```python
from build123d import *

# Parameters (mm, degrees)
F0_W     = 412.75
F0_H     = 295.275
F1_DEPTH = 25.4
F2_W     = 19.05
F2_H     = 387.35
F3_DEPTH = 25.4


with BuildPart() as f1:
    # F0 (on Top) → F1 (new body)
    with BuildSketch(Plane.XY):
        Polygon((279.4, -203.2), (279.4, 203.2), (-279.4, 203.2), (-330.2, 203.2), (-330.2, -203.2), (-279.4, -203.2), align=None)
        Rectangle(F0_W, F0_H, mode=Mode.SUBTRACT)
    extrude(amount=F1_DEPTH)

    # F2 (on face) → F3 (join)
    with BuildSketch(Plane(origin=(0, 0, 0), x_dir=(1, 0, 0), z_dir=(0, 0, -1))):
        Polygon((279.4, 203.2), (-330.2, 203.2), (-330.2, 184.15), (-311.15, 184.15), (260.35, 184.15), (279.4, 184.15), align=None)
        with Locations((269.875, -9.525)):
            Rectangle(F2_W, F2_H)
        with Locations((-320.675, -9.525)):
            Rectangle(F2_W, F2_H)
    extrude(amount=F3_DEPTH)


solid = f1.part
```
CAD build for the part. Positions are in the model's coordinates, mm. A direction names the side the tool comes from. Round coordinates to 2 decimals unless told otherwise and drop trailing zeros. Write each loop counter-clockwise with the first axis right and the second up, starting at its lowest first coordinate (ties: lowest second). Pieces come first, ordered by that corner, then holes.
Item 1: Band-saw the part on A-A on y = 0.5. Write the cut outline in (x, z) (3 decimals).
Filled in:
outline: (-330.2, -25.4) - (-311.15, -25.4) - (-311.15, 0) - (-206.375, 0) - (-206.375, 25.4) - (-330.2, 25.4) - close; (206.375, 0) - (260.35, 0) - (260.35, -25.4) - (279.4, -25.4) - (279.4, 25.4) - (206.375, 25.4) - close
Item 2: Band-saw the part on B-B on x = 80.5. Write the cut outline in (y, z).
Filled in:
outline: (-203.2, -25.4) - (-184.15, -25.4) - (-184.15, 0) - (-147.64, 0) - (-147.64, 25.4) - (-203.2, 25.4) - close; (147.64, 0) - (203.2, 0) - (203.2, 25.4) - (147.64, 25.4) - close
Item 3: Drill centre lines: L1, parallel to X at y = 132, z = -14.5; L2, parallel to X at y = 80.5, z = 19 (3 decimals); L3, parallel to Y at x = 199, z = 3.5. Where is each one in solid material? Low to high.
Filled in:
L1: x = -330.2 to -311.15, 260.35 to 279.4
L2: x = -330.2 to -206.375, 206.375 to 279.4
L3: y = -203.2 to -147.64, 147.64 to 203.2
Item 4: Drop flat-ended pins along their axis: pin 1 Ø12 at (x, z) = (-264.5, -2) entering from +Y; pin 2 Ø8 at (x, y) = (-246, -53.5) entering from -Z; pin 3 Ø20.5 at (x, z) = (112.5, -14) entering from +Y. Give the stop position or say it passes through.
Filled in:
pin 1: stops at y = 203.2
pin 2: stops at z = 0
pin 3: stops at y = -184.15
Item 5: Band-saw the part on C-C on z = 12. Write the cut outline in (x, y) (1 decimal), then the cut area to 3 significant figures.
Filled in:
outline: (-330.2, -203.2) - (279.4, -203.2) - (279.4, 203.2) - (-330.2, 203.2) - close; hole (-206.4, -147.6) - (206.4, -147.6) - (206.4, 147.6) - (-206.4, 147.6) - close
area: 126,000 mm2
Item 6: Tool access for faces 5 (the flat face through (-3, -147.638, 13)), 6 (the flat face through (-30, 203.2, 12)), 7 (the flat face through (-311.15, 12, -13)): list every direction of +Z, -Z, +X, -X, +Y, -Y with a clear straight run to the whole face (end or side of a thin tool).
Filled in:
face 5: +Z, -Z
face 6: +Z, -Z, +X, -X, +Y
face 7: -Z, +Y
Item 7: Band-saw the part on D-D on y = 167. Write the cut outline in (x, z), then the cut area to 3 significant figures.
Filled in:
outline: (-330.2, -25.4) - (-311.15, -25.4) - (-311.15, 0) - (260.35, 0) - (260.35, -25.4) - (279.4, -25.4) - (279.4, 25.4) - (-330.2, 25.4) - close
area: 16,500 mm2
Item 8: Mould opens along Y. For faces 1 (the flat face through (-21, -203.2, 0)), 2 (the flat face through (206.375, -2, 13)), 3 (the flat face through (-29, -184.15, -13)), 4 (the flat face through (260.35, 12, -13)) say: released by +Y, released by -Y, zero draft, split by the parting line, or undercut.
Filled in:
face 1: released by -Y
face 2: undercut
face 3: released by +Y
face 4: zero draft
